from build123d import *

# Parameters (mm, degrees)
F0_R     = 37.65
F0_R_2   = 33.7
F1_DEPTH = 375
F2_SIZE2 = 0.8038475773
F2_SIZE  = 3
F3_SIZE  = 0.5


with BuildPart() as f1:
    # F0 (on Front) → F1 (new body, symmetric)
    with BuildSketch(Plane.XZ):
        Circle(F0_R)
        Circle(F0_R_2, mode=Mode.SUBTRACT)
    extrude(amount=F1_DEPTH, both=True)

    # F2
    f2_edges = [f1.edges().sort_by_distance(p)[0] for p in [
        (-33.7, -375, 0),
        (-33.7, 375, 0),
    ]]
    f2_side = f1.faces().sort_by_distance((-33.7, 0, 0))[0]
    chamfer(f2_edges, length=F2_SIZE, length2=F2_SIZE2, reference=f2_side)

    # F3
    f3_edges = [f1.edges().sort_by_distance(p)[0] for p in [
        (-37.65, -375, 0),
        (-37.65, 375, 0),
    ]]
    chamfer(f3_edges, length=F3_SIZE)


solid = f1.part
Work out the finished part from the listing and answer in its coordinate system (mm). Coordinates: 2 decimals unless noted, no trailing zeros. Write each loop counter-clockwise with the first axis right and the second up, starting at its lowest first coordinate (ties: lowest second). Pieces come first, ordered by that corner, then holes. Notation, with made-up numbers: M 14.25,58.25 L 72.25,58.25 A30 ccw 72.25,81.25 Z; hole C 47.25,13 d4. An arc over 180 degrees is marked long. Use one line per item in the form item = value. Start each with the question number.
1. Each of these flat-tipped pins is pushed along its axis until it touches: P1, Ø12, axis at x = 16, z = 18.5, coming from the +Y side; P2, Ø5, axis at x = -6.5, y = 99, coming from the +Z side; P3, Ø2, axis at x = -20, y = -22.5, coming from the -Z side; P4, Ø8, axis at y = 226.5, z = -11.5, coming from the -X side. Where does it stop, or does it pass through?
2. The part is cut by section C-C (y = -36). Give the vertices of the cut face in (x, z), plus the area to 3 significant figures.
3. The mould has two halves that part along Z. Classify faces 1 (the face through (-8.162, -5.243, -36.755)), 2 (the face through (32.19, 372.19, 10.14)), 3 (the face through (11, -375, -33)): released by +Z, released by -Z, zero draft, split by the parting line, or undercut.
4. The part is cut by section A-A (x = 0). Give the vertices of the cut face in (y, z).
5. The part is cut by section B-B (z = 0). Give the vertices of the cut face in (x, y).
6. Straight lines are drawn through the part: probe 1 along Z at (x, y) = (0, -15); probe 2 along X at (y, z) = (21.5, -3); probe 3 along X at (y, z) = (103.5, -8.5). For each, find the intervals that lie inside material, in ascending order. Write a range as from..to.
Evaluation:
q1.P1 = through
q1.P2 = 37.44
q1.P3 = -32.5
q1.P4 = -36.9
q2.outline = C 0,0 d75.3; hole C 0,0 d67.4
q2.area = 885 mm^2
q3.face_1 = split by the parting line
q3.face_2 = undercut
q3.face_3 = zero draft
q4.outline = M -375,-37.15 L -374.5,-37.65 L 374.5,-37.65 L 375,-37.15 L 375,-34.5 L 372,-33.7 L -372,-33.7 L -375,-34.5 Z; M -375,34.5 L -372,33.7 L 372,33.7 L 375,34.5 L 375,37.15 L 374.5,37.65 L -374.5,37.65 L -375,37.15 Z
q5.outline = M -37.65,-374.5 L -37.15,-375 L -34.5,-375 L -33.7,-372 L -33.7,372 L -34.5,375 L -37.15,375 L -37.65,374.5 Z; M 33.7,-372 L 34.5,-375 L 37.15,-375 L 37.65,-374.5 L 37.65,374.5 L 37.15,375 L 34.5,375 L 33.7,372 Z
q6.probe_1 = -37.65..-33.7, 33.7..37.65
q6.probe_2 = -37.53..-33.57, 33.57..37.53
q6.probe_3 = -36.68..-32.61, 32.61..36.68
